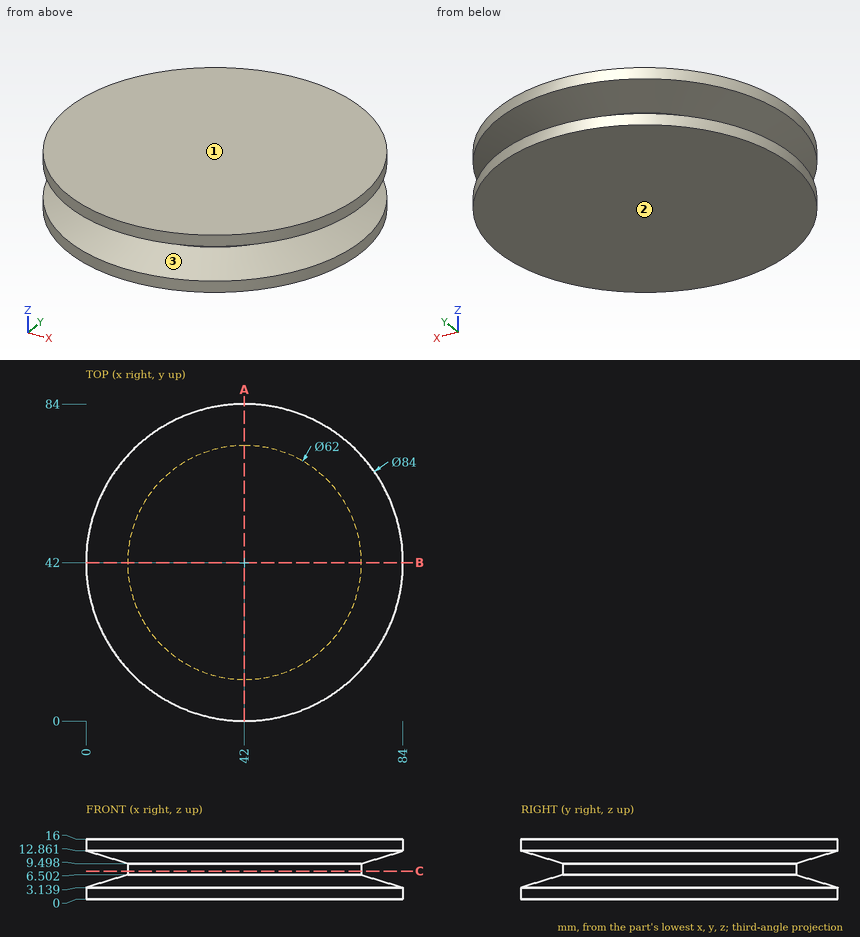
Input: dimensioned drawing with shaded views. Units: mm. Origin: part minimum x, y, z. Coordinates: 2 decimals unless noted, no trailing zeros. Loops run counter-clockwise (first coordinate to the right, second up) from the corner with the lowest first, then second, coordinate; pieces in that order, holes last. Notation, with made-up numbers: (83.25, 12.5) - (111.25, 12.5) arc R26 ccw to (111.25, 47.5) - close; hole circle Ø4 at (25.25, 55). An arc over 180 degrees is marked (long way). One line per question, with ' | ' between items. Start each with the question number.
(1) Cut plane C-C on z = 7.5. Output: boundary loops of the cut face in (x, y).
(2) Draft query along Z for the marked faces 1, 2 and 3. Return one class per face: +Z half, -Z half, draft (parallel to the pull), parting line (faces both ways), or undercut.
(3) Cut plane A-A on x = 42. Output: boundary loops of the cut face in (y, z).
(4) First-contact query: pin 1 (1.5 mm diameter, centred on y = 62.5, z = 12.5, fed in from +X); pin 2 (4 mm diameter, centred on y = 37, z = 3, fed in from -X); pin 3 (1.5 mm diameter, centred on x = 12.5, z = 13, fed in from +Y). Flat tips, straight axial feed; report the tip coordinate or a pass-through.
(5) Ray query, L1, parallel to Z at x = 10, y = 25; L2, parallel to Z at x = 52, y = 77.5; L3, parallel to Y at x = 55, z = 15. Return the intervals inside material, ascending. Write a range as from..to.
Here are the results:
1) outline: circle Ø62 at (42, 42)
2) face 1: +Z half | face 2: -Z half | face 3: undercut
3) outline: (0, 0) - (84, 0) - (84, 3.14) - (73, 6.5) - (73, 9.5) - (84, 12.86) - (84, 16) - (0, 16) - (0, 12.86) - (11, 9.5) - (11, 6.5) - (0, 3.14) - close
4) pin 1: x = 79.02 | pin 2: x = 0.11 | pin 3: y = 72.62
5) L1: 0..4.9, 11.1..16 | L2: 0..4.7, 11.3..16 | L3: 2.06..81.94
